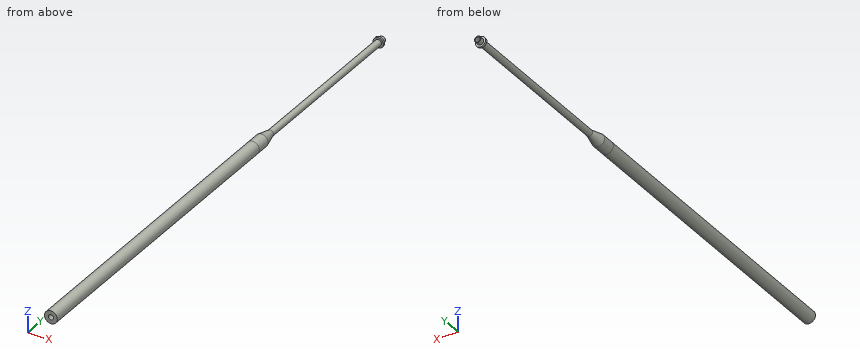
```python
from build123d import *

# Parameters (mm, degrees)
ESQUISSE1_R             = 5
BOSS_EXTRU_1_DEPTH      = 820
ESQUISSE2_R             = 10
BOSS_EXTRU_2_DEPTH      = 500
CHANFREIN1_SIZE         = 10
CHANFREIN1_SIZE_2       = 43.314758743
ESQUISSE3_R             = 4
ENL_V_MAT_EXTRU_1_DEPTH = 821.121942153
ESQUISSE4_R             = 8
ESQUISSE4_R_2           = 4.5
BOSS_EXTRU_3_DEPTH      = 3


with BuildPart() as part:
    # Esquisse1 → Boss.-Extru.1 (new body)
    with BuildSketch(Plane(origin=(0, 0, 0), x_dir=(1, 0, 0), z_dir=(0, 1, 0))):
        with Locations(Location((0, 0, 0), (0, 0, 270))):
            Circle(ESQUISSE1_R)
    extrude(amount=BOSS_EXTRU_1_DEPTH)

    # Esquisse2 → Boss.-Extru.2 (add)
    with BuildSketch(Plane(origin=(0, 0, 0), x_dir=(1, 0, 0), z_dir=(0, 1, 0))):
        with Locations(Location((0, 0, 0), (0, 0, 270))):
            Circle(ESQUISSE2_R)
    extrude(amount=BOSS_EXTRU_2_DEPTH)

    # Chanfrein1
    # the kernel refuses this chamfer: 43.314758743, 10 mm, written as the material it adds along each edge
    with BuildSketch(Plane(origin=(0, 500, 0), x_dir=(0, 0, 1), z_dir=(1, 0, 0))) as chanfrein1_piece_1_section:
        Polygon((5 + CHANFREIN1_SIZE, 0), (5, -CHANFREIN1_SIZE_2), (5, 0), align=None)
    chanfrein1_piece_1 = revolve(axis=Axis((0, 500, 0), (0, -1, 0)), mode=Mode.PRIVATE)
    chanfrein1_piece_1 = chanfrein1_piece_1 & Plane(origin=(0, 533.283833366, 0), x_dir=(0, 0, 1), z_dir=(0, -1, 0)) * Cylinder(10, 174, mode=Mode.PRIVATE)
    add(chanfrein1_piece_1)

    # Esquisse3 → Enlèv. mat.-Extru.1 (cut, through all)
    with BuildSketch(Plane(origin=(0, 820, 0), x_dir=(1, 0, 0), z_dir=(0, 1, 0))):
        with Locations(Location((0, 0, 0), (0, 0, 270))):
            Circle(ESQUISSE3_R)
    extrude(amount=-ENL_V_MAT_EXTRU_1_DEPTH, mode=Mode.SUBTRACT)

    # Esquisse4 → Boss.-Extru.3 (add)
    with BuildSketch(Plane(origin=(0, 810, 0), x_dir=(1, 0, 0), z_dir=(0, 1, 0))):
        with Locations(Location((0, 0, 0), (0, 0, 270))):
            Circle(ESQUISSE4_R)
        Circle(ESQUISSE4_R_2, mode=Mode.SUBTRACT)
    extrude(amount=BOSS_EXTRU_3_DEPTH)


solid = part.part
```
Work out the finished part from the listing and answer in its coordinate system (mm). Give positions to 0.01 mm unless a question says otherwise; leave off trailing zeros. Loops run counter-clockwise (first coordinate to the right, second up) from the corner with the lowest first, then second, coordinate; pieces in that order, holes last. Notation, with made-up numbers: (6, 61.25) -> (19, 61.25) arc R17 cw to (19, 76.25) -> close; hole circle Ø8 at (45, -24). An arc over 180 degrees is marked (long way). Use CSV: the item, a comma, the result in double quotes.
1. Straight lines are drawn through the part: line 1 (X direction, y = 587, z = 0); line 2 (X direction, y = 436, z = 0); line 3 (X direction, y = 321.5, z = 6). For each, find the intervals that lie inside material, in ascending order.
Found:
line 1,"-5 to -4, 4 to 5"
line 2,"-10 to -4, 4 to 10"
line 3,"-8 to 8"
2. The part is cut by section B-B (z = 0). Write down the section's boundary in (x, y).
Found:
outline,"(-10, 0) -> (-4, 0) -> (-4, 820) -> (-5, 820) -> (-5, 813) -> (-8, 813) -> (-8, 810) -> (-5, 810) -> (-5, 543.31) -> (-10, 521.66) -> close; (4, 0) -> (10, 0) -> (10, 521.66) -> (5, 543.31) -> (5, 810) -> (8, 810) -> (8, 813) -> (5, 813) -> (5, 820) -> (4, 820) -> close"
3. Flat-ended cylindrical pins translate along their axes: pin 1 Ø10 at (y, z) = (429, 8) entering from +X; pin 2 Ø3 at (y, z) = (549.5, 6) entering from +X; pin 3 Ø3 at (y, z) = (543, -5.5) entering from -X. Find the tip coordinate at first contact, or state that the pin passes through.
Found:
pin 1,"x = 9.54"
pin 2,"x = 2.18"
pin 3,"x = -3.2"
4. The part is cut by section C-C (y = 232.5). Write down the section's boundary in (x, z), then the cut area to 3 significant figures.
Found:
outline,"circle Ø20 at (0, 0); hole circle Ø8 at (0, 0)"
area,"264 mm^2"
5. The part is cut by section A-A (x = 0). Write down the section's boundary in (y, z), then the cut area to 3 significant figures.
Found:
outline,"(0, -10) -> (521.66, -10) -> (543.31, -5) -> (810, -5) -> (810, -8) -> (813, -8) -> (813, -5) -> (820, -5) -> (820, -4) -> (0, -4) -> close; (0, 4) -> (820, 4) -> (820, 5) -> (813, 5) -> (813, 8) -> (810, 8) -> (810, 5) -> (543.31, 5) -> (521.66, 10) -> (0, 10) -> close"
area,"6,980 mm^2"
6. The part is cut by section D-D (y = 560). Write down the section's boundary in (x, z).
Found:
outline,"circle Ø10 at (0, 0); hole circle Ø8 at (0, 0)"
